The listing builds one solid part. Answer for the finished solid, in the listing's coordinates (mm). A direction names the side the tool comes from. Give positions to 0.01 mm unless a question says otherwise; leave off trailing zeros. Write each loop counter-clockwise with the first axis right and the second up, starting at its lowest first coordinate (ties: lowest second). Pieces come first, ordered by that corner, then holes. Notation, with made-up numbers: (72, -22) -> (84, -22) arc R19 cw to (84, -7) -> close; hole circle Ø8 at (2, -8). An arc over 180 degrees is marked (long way). Put each result on its own line as item: value. Start each with the question number.
1) A cutting plane is placed at A-A (y = 0). Write down the section's boundary in (x, z), then the cut area to 3 significant figures.
2) A cutting plane is placed at D-D (x = 38). Write down the section's boundary in (y, z), then the cut area to 3 significant figures.
3) A cutting plane is placed at C-C (x = 5.5). Write down the section's boundary in (y, z), then the cut area to 3 significant figures.
4) Find the intervals of material crossed by line 1 along X through (y, z) = (-21, 4.15); line 2 along Y through (x, z) = (48.5, 2.65); line 3 along Y through (x, z) = (0, 3.9), in increasing order. Write a range as from..to.
5) For a pull along Y with two mould halves and no side action, classify faces 4 (the cylindrical face through (54.5, -19.55, 2.46)), 5 (the flat face through (-34, 24, 2)), 6 (the flat face through (41, -20, 2)) as released by +Y, released by -Y, zero draft, split by the parting line, or undercut.
6) For faces 1 (the flat face through (41, 20, 2)), 2 (the flat face through (-34, -24, 2)), 3 (the flat face through (37, -3, 5)), determine the directions among +Z, -Z, +X, -X, +Y, -Y from which every point of the face is accessible in a straight line to the end or side of a thin tool.
7) Flat-ended cylindrical pins translate along their axes: pin 1 Ø2.5 at (x, y) = (-36.93, 20) entering from +Z; pin 2 Ø1.5 at (y, z) = (4, 2) entering from +X; pin 3 Ø2.5 at (x, z) = (-33.5, 3.5) entering from +Y; pin 4 Ø2.5 at (x, z) = (-32.5, 2.5) entering from -Y. Find the tip coordinate at first contact, or state that the pin passes through.
8) A cutting plane is placed at B-B (z = 3.15). Write down the section's boundary in (x, y).
from build123d import *

# Parameters (mm, degrees)
SKETCH1_R           = 1.5
SKETCH1_R_2         = 35
BOSS_EXTRUDE1_DEPTH = 5


with BuildPart() as part:
    # Sketch1 → Boss-Extrude1 (new body)
    with BuildSketch(Plane.XY):
        with BuildLine():
            Line((-30.740852298, 24), (-36.932370625, 24))
            ThreePointArc((-36.932370625, 24), (-40.932370625, 20), (-36.932370625, 16))
            Line((-36.932370625, 16), (-37.002837962, 12.320307738))
            ThreePointArc((-37.002837962, 12.320307738), (-38.941537608, -2.134630811), (-35.434469198, -16.291052533))
            ThreePointArc((-35.434469198, -16.291052533), (-40.858933363, -19.237041898), (-36.932370625, -24))
            Line((-36.932370625, -24), (-30.740852298, -24))
            ThreePointArc((-30.740852298, -24), (2.424369111, -38.924573657), (33.481338086, -20))
            Line((33.481338086, -20), (49.067629375, -20))
            ThreePointArc((49.067629375, -20), (55.8960565, -22.828427125), (53.067629375, -16))
            Line((53.067629375, -16), (53.067629375, 16))
            ThreePointArc((53.067629375, 16), (55.8960565, 22.828427125), (49.067629375, 20))
            Line((49.067629375, 20), (33.481338086, 20))
            ThreePointArc((33.481338086, 20), (2.424369111, 38.924573657), (-30.740852298, 24))
        make_face()
        with Locations((-36.932370625, -20)):
            Circle(SKETCH1_R, mode=Mode.SUBTRACT)
        with Locations((53.067629375, -20)):
            Circle(SKETCH1_R, mode=Mode.SUBTRACT)
        Circle(SKETCH1_R_2, mode=Mode.SUBTRACT)
        with Locations((-36.932370625, 20)):
            Circle(SKETCH1_R, mode=Mode.SUBTRACT)
        with Locations((53.067629375, 20)):
            Circle(SKETCH1_R, mode=Mode.SUBTRACT)
    extrude(amount=BOSS_EXTRUDE1_DEPTH)


solid = part.part
Reply:
1. outline: (-39, 0) -> (-35, 0) -> (-35, 5) -> (-39, 5) -> close; (35, 0) -> (53.07, 0) -> (53.07, 5) -> (35, 5) -> close
1. area: 110 mm2
2. outline: (-20, 0) -> (20, 0) -> (20, 5) -> (-20, 5) -> close
2. area: 200 mm2
3. outline: (-38.61, 0) -> (-34.57, 0) -> (-34.57, 5) -> (-38.61, 5) -> close; (34.57, 0) -> (38.61, 0) -> (38.61, 5) -> (34.57, 5) -> close
3. area: 40.5 mm2
4. line 1: x = -40.81..-38.05, -35.81..-28, 28..32.86, 49.19..51.95, 54.19..56.94
4. line 2: y = -20..20
4. line 3: y = -39..-35, 35..39
5. face 4: undercut
5. face 5: released by +Y
5. face 6: released by -Y
6. face 1: +Z, -Z, +Y
6. face 2: +Z, -Z, -X, -Y
6. face 3: +Z, +X, -X, +Y, -Y
7. pin 1: passes through
7. pin 2: stops at x = 53.07
7. pin 3: stops at y = 24
7. pin 4: stops at y = -24
8. outline: (-37, 12.32) arc R39 ccw to (-35.43, -16.29) arc R4 ccw (long way) to (-36.93, -24) -> (-30.74, -24) arc R39 ccw to (33.48, -20) -> (49.07, -20) arc R4 ccw (long way) to (53.07, -16) -> (53.07, 16) arc R4 ccw (long way) to (49.07, 20) -> (33.48, 20) arc R39 ccw to (-30.74, 24) -> (-36.93, 24) arc R4 ccw to (-36.93, 16) -> close; hole circle Ø3 at (-36.93, -20); hole circle Ø3 at (-36.93, 20); hole circle Ø70 at (0, 0); hole circle Ø3 at (53.07, -20); hole circle Ø3 at (53.07, 20)
